Design review of the part built by this model. Coordinates are the model's own, in mm. Face numbers are marked on the shaded views. A direction names the side the tool comes from. Round coordinates to 2 decimals unless told otherwise and drop trailing zeros. Order: outer loops, then holes, each group sorted by start corner. A loop starts at its lowest first (then second) coordinate and runs counter-clockwise, first axis right, second up. Notation, with made-up numbers: (31.25, 88) - (87.25, 88) arc R22 ccw to (87.25, 127) - close; hole circle Ø2 at (8, 3.5). An arc over 180 degrees is marked (long way). Use CSV: the item, a comma, the result in double quotes. Start each with the question number.
from build123d import *

# Parameters (mm, degrees)
BOSS_EXTRUDE1_DEPTH = 130
SHELL1_T            = -4


with BuildPart() as part:
    # Sketch1 → Boss-Extrude1 (new body)
    with BuildSketch(Plane.XY):
        Polygon((-304.073172001, 21.586402266), (5.926827999, -233.413597734), (375.926827999, -233.413597734), (375.926827999, 141.586402266), (-304.073172001, 141.586402266), align=None)
    extrude(amount=BOSS_EXTRUDE1_DEPTH)

    # Shell1
    shell1_openings = [part.faces().sort_by_distance(p)[0] for p in [
        (35.926827999, 141.586402266, 65),
    ]]
    offset(amount=SHELL1_T, openings=shell1_openings, kind=Kind.INTERSECTION)


solid = part.part
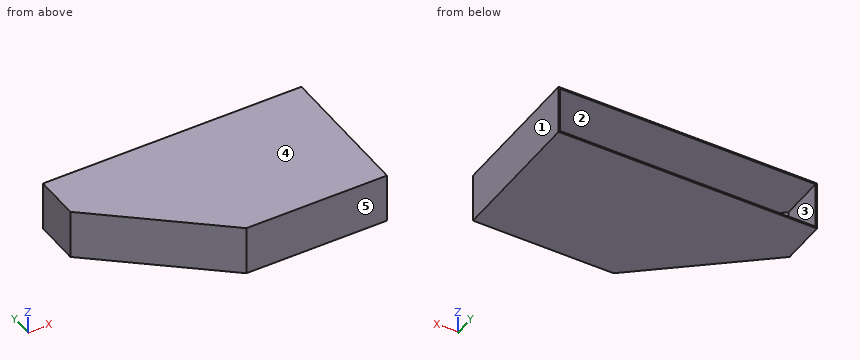
Q1. Tool access review of the marked faces 1 and 2: name each direction out of +Z, -Z, +X, -X, +Y, -Y from which nothing blocks a thin tool from reaching the whole face with its end or side.
Q2. Take a section at A-A (y = 30). State the section outline as (x, z) points.
Q3. Take a section at B-B (z = 76.5). State the section outline as (x, y) points, plus the area to 3 significant figures.
Q4. Take a section at C-C (x = 223.5). State the section outline as (y, z) points, plus the area to 3 significant figures.
Q5. The part is to be moulded in two halves that separate along Z. For the marked faces 3, 4 and 5, say which applies: +Z half, -Z half, draft (parallel to the pull), parting line (faces both ways), or undercut.
Q6. Take a section at D-D (y = -95.5). State the section outline as (x, z) points, plus the area to 3 significant figures.
Q7. Clearance check with a flat-ended pin moving along its axis: pin 1 (4 mm diameter, centred on x = -101.5, z = 31.5, fed in from +Y). State where the tip first meets the part, or that it passes through.
Q8. For L1, parallel to Z at x = 218, y = -83; L2, parallel to X at y = 66.5, z = 35; L3, parallel to Y at x = 188.5, z = 89, list the stretches that pass through material, from the lowest coordinate up. Write a range as [from, to].
Findings below:
1,face 1,"+Z, -Z, +X, +Y, -Y"
1,face 2,"+Y"
2,outline,"(-304.07, 0) - (375.93, 0) - (375.93, 130) - (-304.07, 130) - close; hole (-300.07, 4) - (371.93, 4) - (371.93, 126) - (-300.07, 126) - close"
3,outline,"(-304.07, 21.59) - (5.93, -233.41) - (375.93, -233.41) - (375.93, 141.59) - (371.93, 141.59) - (371.93, -229.41) - (7.36, -229.41) - (-300.07, 23.48) - (-300.07, 141.59) - (-304.07, 141.59) - close"
3,area,"5,040 mm^2"
4,outline,"(-233.41, 0) - (141.59, 0) - (141.59, 4) - (-229.41, 4) - (-229.41, 126) - (141.59, 126) - (141.59, 130) - (-233.41, 130) - close"
4,area,"3,490 mm^2"
5,face 3,"undercut"
5,face 4,"+Z half"
5,face 5,"draft"
6,outline,"(-161.73, 0) - (375.93, 0) - (375.93, 130) - (-161.73, 130) - close; hole (-155.44, 4) - (371.93, 4) - (371.93, 126) - (-155.44, 126) - close"
6,area,"5,560 mm^2"
7,pin 1,"stops at y = -138.22"
8,L1,"z = [0, 4], [126, 130]"
8,L2,"x = [-304.07, -300.07], [371.93, 375.93]"
8,L3,"y = [-233.41, -229.41]"
